from build123d import *

# Parameters (mm, degrees)
F0_W     = 800
F0_H     = 1000
F1_DEPTH = 10
F2_W     = 680
F2_H     = 120
F2_W_2   = 120
F2_H_2   = 880
F3_DEPTH = 30
F4_W     = 30
F4_H     = 25
F4_H_2   = 130
F5_DEPTH = 680
F6_W     = 18
F6_H     = 20
F7_DEPTH = 680


with BuildPart() as f1:
    # F0 (on Front) → F1 (new body)
    with BuildSketch(Plane.XZ):
        Rectangle(F0_W, F0_H)
    extrude(amount=F1_DEPTH)

    # F2 (on face) → F3 (join)
    with BuildSketch(Plane.XZ.offset(10)):
        with Locations((60, 440)):
            Rectangle(F2_W, F2_H)
        with Locations((-340, -60)):
            Rectangle(F2_W_2, F2_H_2)
        with Locations((-340, 440)):
            Rectangle(F2_W_2, F2_H)
    extrude(amount=F3_DEPTH)

    # F4 (on face) → F5 (join)
    with BuildSketch(Plane.YZ.offset(-280)):
        with Locations((-25, 267.5)):
            Rectangle(F4_W, F4_H)
        with Locations((-25, 142.5)):
            Rectangle(F4_W, F4_H)
        with Locations((-25, 17.5)):
            Rectangle(F4_W, F4_H)
        with Locations((-25, -107.5)):
            Rectangle(F4_W, F4_H)
        with Locations((-25, -232.5)):
            Rectangle(F4_W, F4_H)
        with Locations((-25, -357.5)):
            Rectangle(F4_W, F4_H)
        with Locations((-25, -435)):
            Rectangle(F4_W, F4_H_2)
    extrude(amount=F5_DEPTH)

    # F6 (on face) → F7 (cut)
    with BuildSketch(Plane.YZ.offset(400)):
        with Locations((-19, 270)):
            Rectangle(F6_W, F6_H)
        with Locations((-19, 145)):
            Rectangle(F6_W, F6_H)
        with Locations((-19, 20)):
            Rectangle(F6_W, F6_H)
        with Locations((-19, -105)):
            Rectangle(F6_W, F6_H)
        with Locations((-19, -230)):
            Rectangle(F6_W, F6_H)
        with Locations((-19, -355)):
            Rectangle(F6_W, F6_H)
    extrude(amount=-F7_DEPTH, mode=Mode.SUBTRACT)


solid = f1.part
Could you check a few things on this model? Use its own coordinates, in mm. A direction names the side the tool comes from. Give positions to 0.01 mm unless a question says otherwise; leave off trailing zeros. Write each loop counter-clockwise with the first axis right and the second up, starting at its lowest first coordinate (ties: lowest second). Pieces come first, ordered by that corner, then holes. Notation, with made-up numbers: (41.5, 11) -> (47.5, 11) arc R16 ccw to (47.5, 21) -> close; hole circle Ø4 at (64, 15). An arc over 180 degrees is marked (long way). Write each question's results on one line, items separated by ' | '. Start each with the question number.
Q1. We'd pull the mould along Z, two halves only. Please class faces 4 (the face through (65, -10, -181)), 5 (the face through (65, -28, -230)), 6 (the face through (-400, -20, 7)): +Z half, -Z half, draft (parallel to the pull), parting line (faces both ways), or undercut.
Q2. Suppose I cut it at A-A, the plane y = -17.5. List the corners of the cut face in (x, z) for me, and give its area (3 significant figures).
Q3. Suppose I cut it at B-B, the plane z = 69.5. List the corners of the cut face in (x, y) for me.
Q4. Which directions (+Z, -Z, +X, -X, +Y, -Y) give clear straight access to the entire face, cutting with the end or side of a thin tool? Please do faces 1 (the face through (-6, 0, 7)), 2 (the face through (65, -10, -56)), 3 (the face through (55, -25, 130)).
Q5. I'm going to push a flat-ended pin straight in: pin 1 Ø9 at (y, z) = (-24, -203) entering from +X. Where does the tip first touch, or does it pass through?
Q6. I need wall thicknesses on probe 1 along Y at (x, z) = (150.5, 270); probe 2 along X at (y, z) = (-29, 376.5); probe 3 along Y at (x, z) = (-120, 107). Which ranges of each line are inside material? Lowest first, please.
Outcome:
1) face 4: undercut | face 5: undercut | face 6: draft
2) outline: (-400, -500) -> (400, -500) -> (400, -365) -> (-280, -365) -> (-280, -245) -> (400, -245) -> (400, -240) -> (-280, -240) -> (-280, -120) -> (400, -120) -> (400, -115) -> (-280, -115) -> (-280, 5) -> (400, 5) -> (400, 10) -> (-280, 10) -> (-280, 130) -> (400, 130) -> (400, 135) -> (-280, 135) -> (-280, 255) -> (400, 255) -> (400, 260) -> (-280, 260) -> (-280, 380) -> (400, 380) -> (400, 500) -> (-400, 500) -> close | area: 310,000 mm2
3) outline: (-400, -40) -> (-280, -40) -> (-280, -10) -> (400, -10) -> (400, 0) -> (-400, 0) -> close
4) face 1: +Z, -Z, +X, -X, +Y | face 2: +X | face 3: +X, -Y
5) pin 1: x = -280
6) probe 1: -40 to -28, -10 to 0 | probe 2: -400 to -280 | probe 3: -10 to 0
